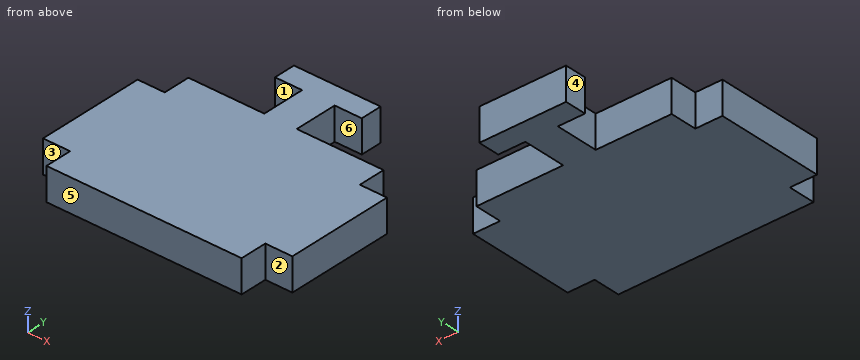
Autodesk Inventor part; units mm, degrees
ref_plane "YZ Plane" through (0, 0, 0) normal (1, 0, 0) x (0, 1, 0)
ref_plane "XZ Plane" through (0, 0, 0) normal (0, 1, 0) x (-1, 0, 0)
ref_plane "XY Plane" through (0, 0, 0) normal (0, 0, 1) x (1, 0, 0)
sketch "Sketch1" plane through (0, 0, 0) normal (0, 0, 1) x (1, 0, 0)
  line L0 (0, 0) -> (18, 0)
  line L1 (18, 0) -> (18, 15)
  line L2 (18, 15) -> (0, 15)
  line L3 (0, 15) -> (0, 0)
  line L4 (20.5, 12.5) -> (18, 12.5)
  line L5 (18, 12.5) -> (18, 2.5)
  line L6 (18, 2.5) -> (20.5, 2.5)
  line L7 (20.5, 2.5) -> (20.5, 12.5)
  line L8 (20.5, 12.5) -> (18, 2.5) construction
  line L9 (18, 12.5) -> (20.5, 2.5) construction
  line L10 (-2.5, 12.5) -> (0, 12.5)
  line L11 (0, 12.5) -> (0, 2.5)
  line L12 (0, 2.5) -> (-2.5, 2.5)
  line L13 (-2.5, 2.5) -> (-2.5, 12.5)
  line L14 (-2.5, 12.5) -> (0, 2.5) construction
  line L15 (0, 12.5) -> (-2.5, 2.5) construction
  line L16 (7, 15) -> (7, 19)
  line L17 (7, 19) -> (4.5, 19)
  line L18 (4.5, 19) -> (4.5, 21)
  line L19 (4.5, 21) -> (12.5, 21)
  line L20 (12.5, 21) -> (12.5, 19)
  line L21 (12.5, 19) -> (10, 19)
  line L22 (10, 19) -> (10, 15)
  point P0 (19.25, 7.5)
  point P1 (-1.25, 7.5)
  point P2 (18, 7.5)
  point P3 (0, 7.5)
  point P4 (0, 12.5)
  dimension "d0" = 18
  dimension "d1" = 15
  dimension "d2" = 2.5
  dimension "d3" = 2.5
  dimension "d4" = 10
  dimension "d5" = 4
  dimension "d6" = 2.5
  dimension "d7" = 2
  dimension "d8" = 8
  dimension "d9" = 2
  dimension "d10" = 2.5
  dimension "d11" = 7
extrude "Extrusion1" add sketch "Sketch1" along normal blind 3
properties part number "Spring_holder"
Model file for the job. Use its own axes, mm. Face numbers are marked on the shaded views. A direction names the side the tool comes from. Coordinates: 2 decimals unless noted, no trailing zeros. Loops run counter-clockwise (first coordinate to the right, second up) from the corner with the lowest first, then second, coordinate; pieces in that order, holes last. Notation, with made-up numbers: (3, 42) - (46, 42) arc R19 ccw to (46, 65) - close; hole circle Ø9 at (87.5, 71.5). An arc over 180 degrees is marked (long way). Answer as a JSON object with one key per item and string values. Group by question number.
(1) Cut at B-B (z = 2.3). Give the cut face in (x, y).
(2) Cut at D-D (x = 14). Give the cut face in (y, z).
(3) Probe line 1 along X through (y, z) = (12.75, 0.95); line 2 along X through (y, z) = (16.5, 2.95); line 3 along Y through (x, z) = (10.25, 2.75). List the from-to ranges inside material, lowest first.
(4) Two-plate mould, pull along Y, no slides. Class the marked faces 4, 5 and 6: released by +Y, released by -Y, zero draft, split by the parting line, or undercut.
(5) Flat gauge pins, fed straight in: pin 1 (1.2 mm diameter, centred on y = 14, z = 2, fed in from -X); pin 2 (1.2 mm diameter, centred on y = 13.5, z = 1.5, fed in from +X); pin 3 (1.5 mm diameter, centred on x = 2.5, z = 1.5, fed in from +Y). Where does each tip first touch, or does it go through?
(6) Tool access for the marked faces 1, 2 and 3: list every direction of +Z, -Z, +X, -X, +Y, -Y with a clear straight run to the whole face (end or side of a thin tool).
(7) Cut at C-C (y = 16.75). Give the cut face in (x, z), then the cut area to 3 significant figures.
(8) Cut at A-A (x = 10.75). Give the cut face in (y, z).
Geometry says:
{
 "1": {"outline": "(-2.5, 2.5) - (0, 2.5) - (0, 0) - (18, 0) - (18, 2.5) - (20.5, 2.5) - (20.5, 12.5) - (18, 12.5) - (18, 15) - (10, 15) - (10, 19) - (12.5, 19) - (12.5, 21) - (4.5, 21) - (4.5, 19) - (7, 19) - (7, 15) - (0, 15) - (0, 12.5) - (-2.5, 12.5) - close"},
 "2": {"outline": "(0, 0) - (15, 0) - (15, 3) - (0, 3) - close"},
 "3": {"line 1": "x = 0 to 18", "line 2": "x = 7 to 10", "line 3": "y = 0 to 15, 19 to 21"},
 "4": {"face 4": "zero draft", "face 5": "released by -Y", "face 6": "undercut"},
 "5": {"pin 1": "stops at x = 0", "pin 2": "stops at x = 18", "pin 3": "stops at y = 15"},
 "6": {"face 1": "+Z, -Z, -X", "face 2": "+Z, -Z, +X, -Y", "face 3": "+Z, -Z, -X, -Y"},
 "7": {"outline": "(7, 0) - (10, 0) - (10, 3) - (7, 3) - close", "area": "9.00 mm^2"},
 "8": {"outline": "(0, 0) - (15, 0) - (15, 3) - (0, 3) - close; (19, 0) - (21, 0) - (21, 3) - (19, 3) - close"}
}
